Can you work these out from the model? Positions are in its coordinate system, mm. Face numbers are marked on the shaded views. A direction names the side the tool comes from. Coordinates: 2 decimals unless noted, no trailing zeros. Order: outer loops, then holes, each group sorted by start corner. A loop starts at its lowest first (then second) coordinate and runs counter-clockwise, first axis right, second up. Notation, with made-up numbers: (72, 57) -> (92, 57) arc R18 ccw to (92, 82) -> close; hole circle Ø3 at (80.25, 15.5). An arc over 180 degrees is marked (long way). Write item = value, one per line.
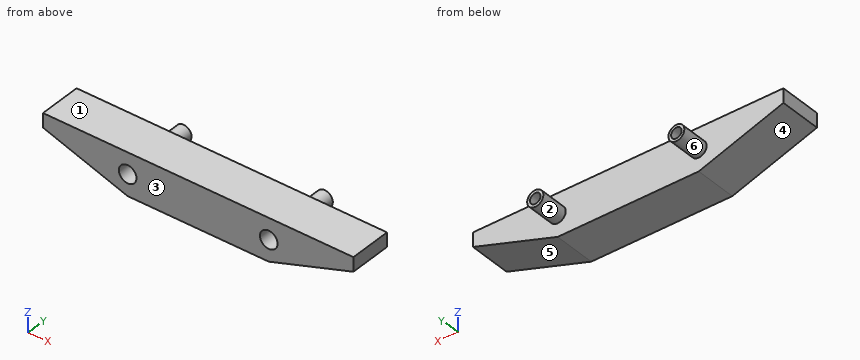
```python
from build123d import *

# Parameters (mm, degrees)
BOSS_EXTRUDE1_DEPTH = 12
SKETCH2_R           = 2.5
CUT_EXTRUDE1_DEPTH  = 5
SKETCH3_R           = 1.5
CUT_EXTRUDE2_DEPTH  = 90.089842294
SKETCH4_R           = 2.25
SKETCH4_R_2         = 1.5
SKETCH4_R_3         = 2.294622505
BOSS_EXTRUDE2_DEPTH = 8


with BuildPart() as part:
    # Sketch1 → Boss-Extrude1 (new body)
    with BuildSketch(Plane(origin=(0, 0, 0), x_dir=(1, 0, 0), z_dir=(0, 1, 0))):
        Polygon((0, 0), (88, 0), (88, 4), (64, 12), (24, 12), (0, 4), align=None)
    extrude(amount=BOSS_EXTRUDE1_DEPTH)

    # Sketch2 → Cut-Extrude1 (cut)
    with BuildSketch(Plane(origin=(0, 0, 0), x_dir=(-1, 0, 0), z_dir=(0, -1, 0))):
        with Locations(Location((-24, 6, 0), (0, 0, 90))):
            Circle(SKETCH2_R)
        with Locations(Location((-64, 6, 0), (0, 0, 90))):
            Circle(SKETCH2_R)
    extrude(amount=-CUT_EXTRUDE1_DEPTH, mode=Mode.SUBTRACT)

    # Sketch3 → Cut-Extrude2 (cut, through all)
    with BuildSketch(Plane(origin=(0, 5, 0), x_dir=(-1, 0, 0), z_dir=(0, -1, 0))):
        with Locations(Location((-24, 6, 0), (0, 0, 90))):
            Circle(SKETCH3_R)
        with Locations(Location((-64, 6, 0), (0, 0, 90))):
            Circle(SKETCH3_R)
    extrude(amount=-CUT_EXTRUDE2_DEPTH, mode=Mode.SUBTRACT)

    # Sketch4 → Boss-Extrude2 (add)
    with BuildSketch(Plane(origin=(0, 12, 0), x_dir=(1, 0, 0), z_dir=(0, 1, 0))):
        with Locations(Location((24, 6, 0), (0, 0, 270))):
            Circle(SKETCH4_R)
        with Locations(Location((24, 6, 0), (0, 0, 90))):
            Circle(SKETCH4_R_2, mode=Mode.SUBTRACT)
        with Locations(Location((64, 6, 0), (0, 0, 270))):
            Circle(SKETCH4_R_3)
        with Locations(Location((64, 6, 0), (0, 0, 90))):
            Circle(SKETCH4_R_2, mode=Mode.SUBTRACT)
    extrude(amount=BOSS_EXTRUDE2_DEPTH)


solid = part.part
```
Item 1: For the marked faces 1 and 2, which set-ups out of +Z, -Z, +X, -X, +Y, -Y let a thin tool reach every point of the face, with its end or its side?
A:
face_1 = +Z, +X, -X, +Y, -Y
face_2 = +Y
Item 2: I want a section at C-C, the plane x = 73. Please give me the cut outline in (y, z).
A:
outline = (0, -9) -> (12, -9) -> (12, 0) -> (0, 0) -> close
Item 3: I want a section at B-B, the plane y = 10.75. Please give me the cut outline in (x, z), plus the area to 3 significant figures.
A:
outline = (0, -4) -> (24, -12) -> (64, -12) -> (88, -4) -> (88, 0) -> (0, 0) -> close; hole circle Ø3 at (24, -6); hole circle Ø3 at (64, -6)
area = 850 mm2
Item 4: I want a section at A-A, the plane z = -6. Please give me the cut outline in (x, y).
A:
outline = (6, 0) -> (21.5, 0) -> (21.5, 5) -> (22.5, 5) -> (22.5, 20) -> (21.75, 20) -> (21.75, 12) -> (6, 12) -> close; (25.5, 5) -> (26.5, 5) -> (26.5, 0) -> (61.5, 0) -> (61.5, 5) -> (62.5, 5) -> (62.5, 20) -> (61.71, 20) -> (61.71, 12) -> (26.25, 12) -> (26.25, 20) -> (25.5, 20) -> close; (65.5, 5) -> (66.5, 5) -> (66.5, 0) -> (82, 0) -> (82, 12) -> (66.29, 12) -> (66.29, 20) -> (65.5, 20) -> close
Item 5: I'm going to push flat-ended pins straight in: P1, Ø4, axis at x = 64.5, z = -7, coming from the -Y side; P2, Ø1, axis at x = 62.5, y = 13, coming from the +Z side; P3, Ø6, axis at x = 49.5, z = -4, coming from the +Y side; P4, Ø1.5, axis at x = 24, z = -5, coming from the -Y side. Where does each tip first touch, or does it pass through?
A:
P1 = 0
P2 = -3.93
P3 = 12
P4 = 5
Item 6: I want a section at D-D, the plane y = 3.75. Please give me the cut outline in (x, z), plus the area to 3 significant figures.
A:
outline = (0, -4) -> (24, -12) -> (64, -12) -> (88, -4) -> (88, 0) -> (0, 0) -> close; hole circle Ø5 at (24, -6); hole circle Ø5 at (64, -6)
area = 825 mm2
Item 7: If I drill on probe 1 along X at (y, z) = (4.5, -3.75); probe 2 along X at (y, z) = (17, -6); probe 3 along Z at (x, y) = (64, 9.75), over which ranges is the centre line in solid material (lowest first)?
A:
probe_1 = 0 to 22.91, 25.09 to 62.91, 65.09 to 88
probe_2 = 21.75 to 22.5, 25.5 to 26.25, 61.71 to 62.5, 65.5 to 66.29
probe_3 = -12 to -7.5, -4.5 to 0
Item 8: If we mould it in two halves opening along X, with no side actions, what happens to the marked faces 3, 4, 5 and 6? For each: pulls with the +X half, pulls with the -X half, needs draft (parallel to the pull), parting line crosses it, or undercut.
A:
face_3 = needs draft
face_4 = pulls with the -X half
face_5 = pulls with the +X half
face_6 = undercut
